Work out the finished part from the listing and answer in its coordinate system (mm). A direction names the side the tool comes from. Coordinates: 2 decimals unless noted, no trailing zeros. Order: outer loops, then holes, each group sorted by start corner. A loop starts at its lowest first (then second) coordinate and runs counter-clockwise, first axis right, second up. Notation, with made-up numbers: M -21.75,43 L 35.25,43 A6 cw 35.25,50 Z; hole C 51,-29 d6. An arc over 180 degrees is marked long. Write item = value, one per line. Start each with the question number.
Q1. Straight lines are drawn through the part: line 1 along X through (y, z) = (6, 1); line 2 along X through (y, z) = (15.25, -23.5); line 3 along Z through (x, y) = (-26.5, 12.5). For each, find the intervals that lie inside material, in ascending order.
Q2. A tool of negligible diameter and unlimited length cuts with its end or side. For faces 5 (the cylindrical face through (55.123, 9.81, -69.244)), 6 (the flat face through (43, 2.705, 66)), 7 (the flat face through (53.359, 12, -69)), from which of +Z, -Z, +X, -X, +Y, -Y can it reach the whole face along a straight path? Write none if from no direction.
Q3. Find section B-B on z = -30.5. Give the vertices of the cut face in (x, y).
Q4. Find section A-A on x = 18. Give the vertices of the cut face in (y, z), and give its area (3 significant figures).
Q5. Find section D-D on z = -52. Give the vertices of the cut face in (x, y), and give its area (3 significant figures).
Q6. Determine the mould class of faces 1 (the flat face through (56.839, 10, 1)), 2 (the flat face through (53.359, 10, 69.4)), 3 (the flat face through (51, 19.863, 0)), 4 (the flat face through (51, 0, 0)) for opening direction Y: released by +Y, released by -Y, zero draft, split by the parting line, or undercut.
Q7. Find section C-C on x = 43. Give the vertices of the cut face in (y, z), and give its area (3 significant figures).
Q8. Each of these flat-tipped pins is pushed along its axis until it touches: P1, Ø3, axis at y = 8, z = -68.5, coming from the -X side; P2, Ø7, axis at x = 42, y = 8.5, coming from the -Z side; P3, Ø8, axis at x = -17.5, y = 5.5, coming from the +Z side; P4, Ø5, axis at y = 9.93, z = -66.48, coming from the +X side. Where does it stop, or does it pass through?
Autodesk Inventor part; units mm, degrees
ref_plane "Work Plane1" through (53.3591, 0, 73.044) normal (1, 0, 0) x (0, 0, -1)
ref_plane "YZ Plane" through (0, 0, 0) normal (1, 0, 0) x (0, 1, 0)
ref_plane "XZ Plane" through (0, 0, 0) normal (0, 1, 0) x (-1, 0, 0)
sketch "Sketch1" plane through (0, 0, 0) normal (0, 1, 0) x (-1, 0, 0)
  circle A0 centre (0, 0) radius 49.9618
  arc A1 (16.0964, -49.1656) -> (16.0964, 49.1656) centre (0, 0) ccw
  line L0 (-56.8389, 73.044) -> (-56.8388, -73.0441)
  line L1 (-56.8388, 0) -> (0, 0) construction
  line L2 (-56.8389, 73.044) -> (16.0964, 49.1656)
  line L3 (-56.8388, -73.0441) -> (16.0964, -49.1656)
  line L4 (-51.7335, 42.7443) -> (-51.7334, -42.7443) construction
  dimension "d0" = 99.9236
  dimension "d1" = 103.4669
  dimension "d2" = 146.0881
  dimension "d3" = 5.1054
extrude "Extrusion1" add sketch "Sketch1" along normal blind 19.8628
ref_plane "Work Plane1" through (53.3591, 0, 73.044) normal (1, 0, 0) x (0, 0, -1)
sketch "Sketch2" plane through (53.3591, 0, 73.044) normal (1, 0, 0) x (0, 0, -1)
  line L0 (146.0881, 0) -> (146.0881, 19.8628) construction
  line L1 (146.0881, 19.8628) -> (122.2096, 19.8628) construction
  line L2 (146.0881, 0) -> (122.2096, 0) construction
  line L3 (23.8785, 19.8628) -> (0, 19.8628) construction
  line L4 (23.8785, 0) -> (0, 0) construction
  line L5 (0, 0) -> (0, 19.8628) construction
  line L6 (23.8785, 0) -> (23.8785, 19.8628) construction
  line L7 (122.2096, 0) -> (122.2096, 19.8628) construction
  line L8 (146.0881, 17.1577) -> (135.763, 17.1577)
  line L9 (135.763, 17.1577) -> (135.763, 2.7051)
  line L10 (135.763, 2.7051) -> (146.0881, 2.7051)
  line L11 (146.0881, 2.7051) -> (146.0881, 17.1577)
  line L12 (0, 17.1577) -> (10.3251, 17.1577)
  line L13 (10.3251, 17.1577) -> (10.3251, 2.7051)
  line L14 (10.3251, 2.7051) -> (0, 2.7051)
  line L15 (0, 2.7051) -> (0, 17.1577)
  point P0 (73.044, 0)
  dimension "d7" = 2.7051
  dimension "d8" = 2.7051
  dimension "d19" = 10.3251
extrude "Extrusion2" cut sketch "Sketch2" against normal blind 76.2
sketch "Sketch3" plane through (53.3591, 0, 73.044) normal (1, 0, 0) x (0, 0, -1)
  line L0 (139.5285, 9.9314) -> (6.5596, 9.9314) construction
  line L1 (73.044, 0) -> (73.044, 9.9314) construction
  line L2 (135.763, 17.1577) -> (135.763, 2.7051) construction
  line L3 (144.9488, 17.1577) -> (135.763, 17.1577) construction
  line L4 (10.3251, 17.1577) -> (1.1393, 17.1577) construction
  line L5 (144.9488, 17.1577) -> (135.763, 17.1577) construction
  point P0 (73.044, 4.9657)
  point P1 (135.763, 9.9314)
  dimension "Cap_Mount_Hole_Spacing" = 132.969
hole "Hole1" at (53.359, 9.9314, -66.4845) at (53.3591, 9.9314, 66.4845) direction (1, 0, 0) diameter 5.5245 end through all
equation "\"d0\" = Diameter"
equation "\"d8\" = d7"
properties part number "Cap_Mount" material "Polycarbonate, Clear"
Findings below:
q1.line_1 = -51.72 to -49.95, 49.95 to 56.84
q1.line_2 = -46.09 to -44.09, 44.09 to 56.84
q1.line_3 = -44.43 to -42.35, 42.35 to 44.43
q2.face_5 = +X, -X
q2.face_6 = +Z, -X
q2.face_7 = -Z, -X
q3.outline = M -41.79,0 L -39.57,0 L -39.57,19.86 L -41.79,19.86 Z; M 39.57,0 L 56.84,0 L 56.84,19.86 L 39.57,19.86 Z
q4.outline = M 0,-60.33 L 19.86,-60.33 L 19.86,-46.61 L 0,-46.61 Z; M 0,46.61 L 19.86,46.61 L 19.86,60.33 L 0,60.33 Z
q4.area = 545 mm^2
q5.outline = M -7.44,0 L 56.84,0 L 56.84,19.86 L -7.44,19.86 Z
q5.area = 1,280 mm^2
q6.face_1 = zero draft
q6.face_2 = undercut
q6.face_3 = released by +Y
q6.face_4 = released by -Y
q7.outline = M 0,-68.51 L 2.71,-68.51 L 2.71,-62.72 L 17.16,-62.72 L 17.16,-68.51 L 19.86,-68.51 L 19.86,-25.44 L 0,-25.44 Z; M 0,25.44 L 19.86,25.44 L 19.86,68.51 L 17.16,68.51 L 17.16,62.72 L 2.71,62.72 L 2.71,68.51 L 0,68.51 Z
q7.area = 1,540 mm^2
q8.P1 = 53.36
q8.P2 = -62.72
q8.P3 = 50.02
q8.P4 = through
